Job drawing, mm, ordinate dimensions from the low corner. One solid piece. Round coordinates to 2 decimals unless told otherwise and drop trailing zeros. Write each loop counter-clockwise with the first axis right and the second up, starting at its lowest first coordinate (ties: lowest second). Pieces come first, ordered by that corner, then holes.
1) Saw through at D-D (x = 15). Write the cut outline in (y, z), plus the area to 3 significant figures.
2) Saw through at C-C (y = 3.75). Write the cut outline in (x, z), plus the area to 3 significant figures.
3) Wall check: probe 1 along Z at (x, y) = (85, 3.75); probe 2 along Z at (x, y) = (50, 7); probe 3 along Z at (x, y) = (12.5, 2.75). Give the ranges that are in metal, low to high.
4) Pull direction Z, two halves, no side cores. Call the marked faces 1, 2 and 3: +Z half, -Z half, draft (parallel to the pull), parting line (faces both ways), or undercut.
5) Saw through at B-B (z = 85). Write the cut outline in (x, y), plus the area to 3 significant figures.
6) Saw through at A-A (x = 50). Write the cut outline in (y, z).
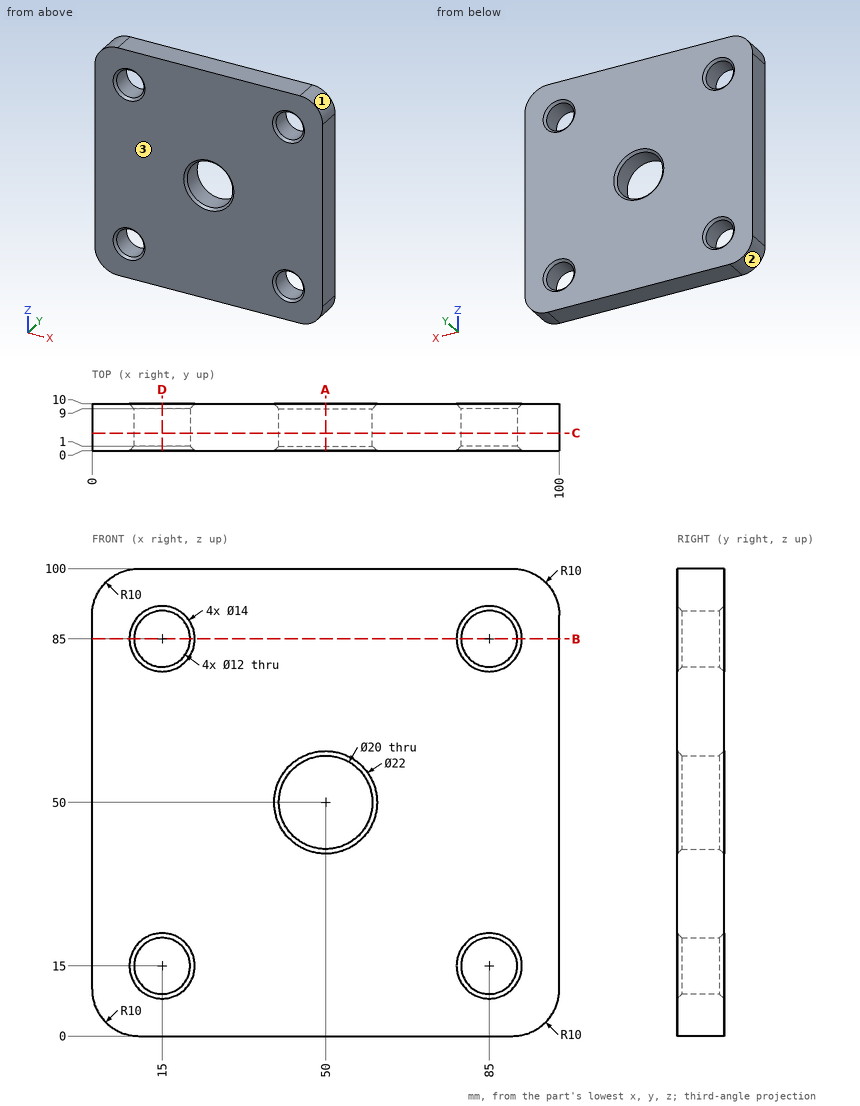
Evaluation:
1. outline: (0, 0) - (10, 0) - (10, 8) - (9, 9) - (1, 9) - (0, 8) - close; (0, 22) - (1, 21) - (9, 21) - (10, 22) - (10, 78) - (9, 79) - (1, 79) - (0, 78) - close; (0, 92) - (1, 91) - (9, 91) - (10, 92) - (10, 100) - (0, 100) - close
1. area: 756 mm2
2. outline: (0, 10) arc R10 ccw to (10, 0) - (90, 0) arc R10 ccw to (100, 10) - (100, 90) arc R10 ccw to (90, 100) - (10, 100) arc R10 ccw to (0, 90) - close; hole circle Ø12 at (15, 15); hole circle Ø12 at (15, 85); hole circle Ø20 at (50, 50); hole circle Ø12 at (85, 15); hole circle Ø12 at (85, 85)
2. area: 9,150 mm2
3. probe 1: z = 0 to 9, 21 to 79, 91 to 100
3. probe 2: z = 0 to 40, 60 to 100
3. probe 3: z = 0 to 9.55, 20.45 to 79.55, 90.45 to 100
4. face 1: +Z half
4. face 2: -Z half
4. face 3: draft
5. outline: (0, 0) - (8, 0) - (9, 1) - (9, 9) - (8, 10) - (0, 10) - close; (21, 1) - (22, 0) - (78, 0) - (79, 1) - (79, 9) - (78, 10) - (22, 10) - (21, 9) - close; (91, 1) - (92, 0) - (100, 0) - (100, 10) - (92, 10) - (91, 9) - close
5. area: 756 mm2
6. outline: (0, 0) - (10, 0) - (10, 39) - (9, 40) - (1, 40) - (0, 39) - close; (0, 61) - (1, 60) - (9, 60) - (10, 61) - (10, 100) - (0, 100) - close
